Source: CAD feature listing. Evaluate the final solid. Frame: model axes, mm. A direction names the side the tool comes from. Give positions to 0.01 mm unless a question says otherwise; leave off trailing zeros. Order: outer loops, then holes, each group sorted by start corner. A loop starts at its lowest first (then second) coordinate and runs counter-clockwise, first axis right, second up. Notation, with made-up numbers: (68, -6) - (123, -6) arc R22 ccw to (123, 23) - close; hole circle Ø6 at (-2.75, 7). An arc over 180 degrees is marked (long way). Answer as CSV lines item,"result".
```python
from build123d import *

# Parameters (mm, degrees)
BOSS_EXTRUDE1_DEPTH      = 10
BOSS_EXTRUDE1_DEPTH_BACK = 10
SKETCH1_W                = 36
SKETCH1_H                = 36
SKETCH2_R                = 12.725
CUT_EXTRUDE1_DEPTH       = 33.372828112
SKETCH5_R                = 4
BOSS_EXTRUDE2_DEPTH      = 25


with BuildPart() as part:
    # Sketch1 → Boss-Extrude1 (new, two sides: drawn at the far end of the back side and taken through both)
    with BuildSketch(Plane(origin=(0, 0, 0), x_dir=(1, 0, 0), z_dir=(0, 1, 0)).offset(-BOSS_EXTRUDE1_DEPTH_BACK)):
        Rectangle(SKETCH1_W, SKETCH1_H)
    extrude(amount=BOSS_EXTRUDE1_DEPTH + BOSS_EXTRUDE1_DEPTH_BACK)

    # Sketch2 → Cut-Extrude1 (cut, through all)
    with BuildSketch(Plane.XZ.offset(10)):
        with Locations(Location((0, 0, 0), (0, 0, 270))):
            Circle(SKETCH2_R)
    extrude(amount=-CUT_EXTRUDE1_DEPTH, mode=Mode.SUBTRACT)

    # Sketch5 → Boss-Extrude2 (add)
    with BuildSketch(Plane(origin=(0, 0, -18), x_dir=(-1, 0, 0), z_dir=(0, 0, -1))):
        Circle(SKETCH5_R)
    boss_extrude2 = extrude(amount=BOSS_EXTRUDE2_DEPTH)

    # Mirror1: Boss-Extrude2 across plane
    add(boss_extrude2.mirror(Plane.XY))


solid = part.part
```
(1) Access query for faces 1 (the flat face through (-12.3, 10, -4.3)), 2 (the cylindrical face through (0.867, -3.905, -30.325)), 3 (the cylindrical face through (0.867, -3.905, 30.325)). Directions: +Z, -Z, +X, -X, +Y, -Y. A direction counts if a zero-diameter tool reaches every point of the face in a straight line with its end or side. Return the directions, or none.
Completed:
face 1,"+Z, -Z, +X, -X, +Y"
face 2,"-Z"
face 3,"+Z"
(2) Cut plane C-C (y = 0). Return loops of the section in (x, z) (3 decimals).
Completed:
outline,"(-18, -18) - (-4, -18) - (-4, -43) - (4, -43) - (4, -18) - (18, -18) - (18, 18) - (4, 18) - (4, 43) - (-4, 43) - (-4, 18) - (-18, 18) - close; hole circle Ø25.45 at (0, 0)"
(3) Cut plane B-B (z = -3). Return loops of the section in (x, y).
Completed:
outline,"(-18, -10) - (-12.37, -10) - (-12.37, 10) - (-18, 10) - close; (12.37, -10) - (18, -10) - (18, 10) - (12.37, 10) - close"
(4) Cut plane D-D (x = 7). Return loops of the section in (y, z), then the cut area to 3 significant figures.
Completed:
outline,"(-10, -18) - (10, -18) - (10, -10.63) - (-10, -10.63) - close; (-10, 10.63) - (10, 10.63) - (10, 18) - (-10, 18) - close"
area,"295 mm²"
(5) Cut plane A-A (x = 0). Return loops of the section in (y, z) (3 decimals), then the cut area to 3 significant figures.
Completed:
outline,"(-10, -18) - (-4, -18) - (-4, -43) - (4, -43) - (4, -18) - (10, -18) - (10, -12.725) - (-10, -12.725) - close; (-10, 12.725) - (10, 12.725) - (10, 18) - (4, 18) - (4, 43) - (-4, 43) - (-4, 18) - (-10, 18) - close"
area,"611 mm²"
(6) Contact query for flat-ended pins moving along their axis: pin 1 (10 mm diameter, centred on x = 14, y = 7.5, fed in from +Z); pin 2 (8 mm diameter, centred on x = -5, z = 0.5, fed in from +Y); pin 3 (8 mm diameter, centred on y = -5, z = -30, fed in from +X); pin 4 (1 mm diameter, centred on x = -14, y = -4.5, fed in from -Z). Output: stop coordinate, or through.
Completed:
pin 1,"z = 18"
pin 2,"through"
pin 3,"x = 3.87"
pin 4,"z = -18"
(7) Mould query, pull axis Z, two halves, no side actions, for faces 4 (the flat face through (-18, 0, 0)), 5 (the cylindrical face through (3.82, -0.14, -12.14)), 6 (the flat face through (0, 0, 43)). Classes: released by +Z, released by -Z, zero draft, split by the parting line, or undercut.
Completed:
face 4,"zero draft"
face 5,"undercut"
face 6,"released by +Z"
(8) Ray query, line 1 (X direction, y = -3.75, z = 0) (3 decimals); line 2 (Z direction, x = 13, y = -4.5); line 3 (Z direction, x = 10, y = -6). Return the intervals inside material, ascending. Write a range as from..to.
Completed:
line 1,"-18..-12.725, 12.725..18"
line 2,"-18..18"
line 3,"-18..-7.87, 7.87..18"
